```python
from build123d import *

# Parameters (mm, degrees)
RESSALTO_EXTRUS_O1_DEPTH = 8
ESBO_O2_R                = 2.4
RESSALTO_EXTRUS_O2_DEPTH = 4


with BuildPart() as part:
    # Esboço1 → Ressalto-extrusão1 (new body)
    with BuildSketch(Plane.XY):
        Polygon((0, 0), (0, 70), (30, 70), (60, 0), align=None)
    extrude(amount=RESSALTO_EXTRUS_O1_DEPTH)

    # Esboço2 → Ressalto-extrusão2 (add)
    with BuildSketch(Plane(origin=(0, 70, 0), x_dir=(1, 0, 0), z_dir=(0, 1, 0))):
        with Locations(Location((25, -4, 0), (0, 0, 90))):
            Circle(ESBO_O2_R)
        with Locations(Location((15, -4, 0), (0, 0, 270))):
            Circle(ESBO_O2_R)
        with Locations(Location((5, -4, 0), (0, 0, 90))):
            Circle(ESBO_O2_R)
    extrude(amount=RESSALTO_EXTRUS_O2_DEPTH)


solid = part.part
```
Build history of the part. All positions in model axes, mm. A direction names the side the tool comes from. Give positions to 0.01 mm unless a question says otherwise; leave off trailing zeros. Loops run counter-clockwise (first coordinate to the right, second up) from the corner with the lowest first, then second, coordinate; pieces in that order, holes last.
1) Drop flat-ended pins along their axis: P1, Ø4, axis at y = 62.5, z = 2.5, coming from the +X side; P2, Ø1.5, axis at x = 11, z = 6, coming from the +Y side; P3, Ø1, axis at y = 26.5, z = 2, coming from the +X side. Give the stop position or say it passes through.
Values follow:
P1: stops at x = 34.07
P2: stops at y = 70
P3: stops at x = 48.86
2) 3-axis set-ups, long thin cutter, end or side, ignore diameter. For faces 4 (the face through (45, 35, 4)), 5 (the face through (27.343, 71.972, 4.52)): which of +Z, -Z, +X, -X, +Y, -Y reach the whole face in a straight line?
Values follow:
face 4: +Z, -Z, +X, +Y
face 5: +Y
3) Two-plate mould, pull along X, no slides. Class faces 1 (the face through (4.28, 71.97, 1.71)), 2 (the face through (0, 35, 4)), 3 (the face through (5, 74, 4)): released by +X, released by -X, zero draft, split by the parting line, or undercut.
Values follow:
face 1: undercut
face 2: released by -X
face 3: zero draft
4) Band-saw the part on B-B on z = 4. List the corners of the cut face in (x, y), then the cut area to 3 significant figures.
Values follow:
outline: (0, 0) - (60, 0) - (30, 70) - (27.4, 70) - (27.4, 74) - (22.6, 74) - (22.6, 70) - (17.4, 70) - (17.4, 74) - (12.6, 74) - (12.6, 70) - (7.4, 70) - (7.4, 74) - (2.6, 74) - (2.6, 70) - (0, 70) - close
area: 3,210 mm2
5) Band-saw the part on D-D on x = 45. List the corners of the cut face in (y, z), then the cut area to 3 significant figures.
Values follow:
outline: (0, 0) - (35, 0) - (35, 8) - (0, 8) - close
area: 280 mm2
6) Band-saw the part on A-A on x = 25. List the corners of the cut face in (y, z).
Values follow:
outline: (0, 0) - (70, 0) - (70, 1.6) - (74, 1.6) - (74, 6.4) - (70, 6.4) - (70, 8) - (0, 8) - close
7) Band-saw the part on C-C on y = 59.5. List the corners of the cut face in (x, z).
Values follow:
outline: (0, 0) - (34.5, 0) - (34.5, 8) - (0, 8) - close
8) Probe line 1 along Y through (x, z) = (12.5, 3.25); line 2 along X through (y, z) = (35.5, 3); line 3 along X through (y, z) = (5.5, 5). List the from-to ranges inside material, lowest first.
Values follow:
line 1: y = 0 to 70
line 2: x = 0 to 44.79
line 3: x = 0 to 57.64
